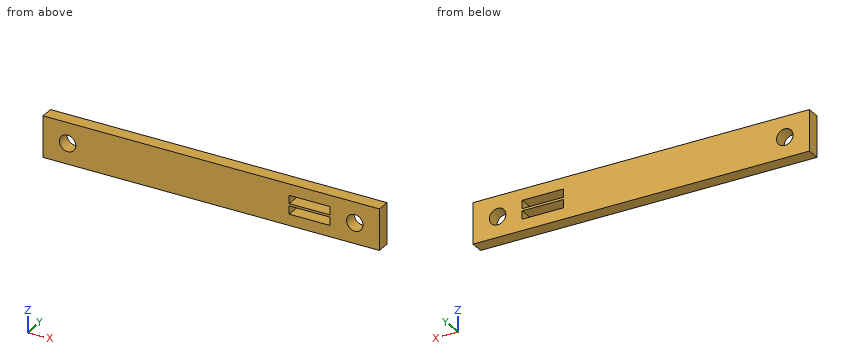
from build123d import *

# Parameters (mm, degrees)
SKETCH1_W           = 41
SKETCH1_H           = 5
SKETCH1_W_2         = 5
SKETCH1_H_2         = 1
SKETCH1_R           = 1
BOSS_EXTRUDE1_DEPTH = 1.6


with BuildPart() as part:
    # Sketch1 → Boss-Extrude1 (new body)
    with BuildSketch(Plane(origin=(0, 0, 0), x_dir=(1, 0, 0), z_dir=(0, 1, 0))):
        with Locations((13.5, 0)):
            Rectangle(SKETCH1_W, SKETCH1_H)
        with Locations((25.5, -0.635)):
            Rectangle(SKETCH1_W_2, SKETCH1_H_2, mode=Mode.SUBTRACT)
        with Locations(Location((-4, 0, 0), (0, 0, 270))):
            Circle(SKETCH1_R, mode=Mode.SUBTRACT)
        with Locations(Location((31, 0, 0), (0, 0, 270))):
            Circle(SKETCH1_R, mode=Mode.SUBTRACT)
        with Locations((25.5, 0.635)):
            Rectangle(SKETCH1_W_2, SKETCH1_H_2, mode=Mode.SUBTRACT)
    extrude(amount=BOSS_EXTRUDE1_DEPTH)


solid = part.part
Read the model definition and answer for the solid it produces. Units are mm, in the model's axes. Round coordinates to 2 decimals unless told otherwise and drop trailing zeros. Write each loop counter-clockwise with the first axis right and the second up, starting at its lowest first coordinate (ties: lowest second). Pieces come first, ordered by that corner, then holes.
Q1. Straight lines are drawn through the part: line 1 (X direction, y = 0.6, z = 0); line 2 (X direction, y = 0.4, z = -1.1); line 3 (X direction, y = 1.2, z = -0.8). For each, find the intervals that lie inside material, in ascending order.
Values:
line 1: x = -7 to -5, -3 to 30, 32 to 34
line 2: x = -7 to 23, 28 to 34
line 3: x = -7 to -4.6, -3.4 to 23, 28 to 30.4, 31.6 to 34
Q2. Find section B-B on y = 0.5. Determine the outline of the cut face in (x, z) (3 decimals), and give its area (3 significant figures).
Values:
outline: (-7, -2.5) - (34, -2.5) - (34, 2.5) - (-7, 2.5) - close; hole circle Ø2 at (-4, 0); hole (23, -1.135) - (28, -1.135) - (28, -0.135) - (23, -0.135) - close; hole (23, 0.135) - (28, 0.135) - (28, 1.135) - (23, 1.135) - close; hole circle Ø2 at (31, 0)
area: 189 mm2
Q3. Find section A-A on x = 31. Determine the outline of the cut face in (y, z).
Values:
outline: (0, -2.5) - (1.6, -2.5) - (1.6, -1) - (0, -1) - close; (0, 1) - (1.6, 1) - (1.6, 2.5) - (0, 2.5) - close
Q4. Flat-ended cylindrical pins translate along their axes: P1, Ø1.5, axis at x = 19.5, z = 1.5, coming from the -Y side; P2, Ø1.2, axis at x = -4, z = 0, coming from the -Y side. Find the tip coordinate at first contact, or state that the pin passes through.
Values:
P1: stops at y = 0
P2: passes through
